Here's how the part is built. I have some questions about the finished solid (model axes, mm). Round coordinates to 2 decimals unless told otherwise and drop trailing zeros. Write each loop counter-clockwise with the first axis right and the second up, starting at its lowest first coordinate (ties: lowest second). Pieces come first, ordered by that corner, then holes. Notation, with made-up numbers: (41, 26.25) - (97, 26.25) arc R22 cw to (97, 50.25) - close; hole circle Ø10 at (-28, 4). An arc over 180 degrees is marked (long way). Return JSON: item names as keys, results as strings. Group by question number.
```python
from build123d import *

# Parameters (mm, degrees)
SKETCH_1_W          = 30
SKETCH_1_H          = 30
EXTRUDE_1_DEPTH     = 10
SKETCH_2_R          = 1.5
CUT_EXTRUDE_1_DEPTH = 11
FILLET_1_R          = 1
SKETCH_3_R          = 14
CUT_EXTRUDE_2_DEPTH = 11


with BuildPart() as part:
    # 草图1 → 凸台-拉伸1 (new body)
    with BuildSketch(Plane(origin=(0, 0, 0), x_dir=(1, 0, 0), z_dir=(0, 1, 0))):
        Rectangle(SKETCH_1_W, SKETCH_1_H)
    extrude(amount=EXTRUDE_1_DEPTH)

    # 草图2 → 切除-拉伸1 (cut, through all)
    with BuildSketch(Plane(origin=(0, 10, 0), x_dir=(1, 0, 0), z_dir=(0, 1, 0))):
        with Locations((-12.3, 12.3)):
            Circle(SKETCH_2_R)
        with Locations((12.3, 12.3)):
            Circle(SKETCH_2_R)
        with Locations((-12.3, -12.3)):
            Circle(SKETCH_2_R)
        with Locations((12.3, -12.3)):
            Circle(SKETCH_2_R)
    extrude(amount=-CUT_EXTRUDE_1_DEPTH, mode=Mode.SUBTRACT)

    # 圆角1
    fillet_1_edges = [part.edges().sort_by_distance(p)[0] for p in [
        (15, 5, 15),
        (-15, 5, 15),
        (-15, 5, -15),
        (15, 5, -15),
    ]]
    fillet(fillet_1_edges, radius=FILLET_1_R)

    # 草图3 → 切除-拉伸2 (cut, through all)
    with BuildSketch(Plane(origin=(0, 10, 0), x_dir=(1, 0, 0), z_dir=(0, 1, 0))):
        Circle(SKETCH_3_R)
    extrude(amount=-CUT_EXTRUDE_2_DEPTH, mode=Mode.SUBTRACT)


solid = part.part
```
1) If we mould it in two halves opening along X, with no side actions, what happens to faces 1 (the cylindrical face through (13.686, 5.07, -11.725)), 2 (the flat face through (0, 5, 15)), 3 (the flat face through (15, 5, 0))? For each: released by +X, released by -X, zero draft, split by the parting line, or undercut.
2) Imagine slicing it at A-A (x = 0). Please give me the cut outline in (y, z).
3) Imagine slicing it at D-D (x = -12.3). Please give me the cut outline in (y, z), plus the area to 3 significant figures.
4) Imagine slicing it at C-C (y = 1.5). Please give me the cut outline in (x, z), plus the area to 3 significant figures.
5) Will this pin go through, and if not, where does the flat tip stop? pin 1 Ø4 at (x, z) = (-12.3, -12.3) entering from +Y.
6) Imagine slicing it at B-B (z = 0). Please give me the cut outline in (x, y).
7) I need wall thicknesses on line 1 along X through (y, z) = (6, -11.75); line 2 along X through (y, z) = (5.5, 12); line 3 along Z through (x, y) = (0, 2.75). Which ranges of each line are inside material? Lowest first, please.
Results found:
{
 "1": {"face 1": "undercut", "face 2": "zero draft", "face 3": "released by +X"},
 "2": {"outline": "(0, -15) - (10, -15) - (10, -14) - (0, -14) - close; (0, 14) - (10, 14) - (10, 15) - (0, 15) - close"},
 "3": {"outline": "(0, -15) - (10, -15) - (10, -13.8) - (0, -13.8) - close; (0, -10.8) - (10, -10.8) - (10, -6.69) - (0, -6.69) - close; (0, 6.69) - (10, 6.69) - (10, 10.8) - (0, 10.8) - close; (0, 13.8) - (10, 13.8) - (10, 15) - (0, 15) - close", "area": "106 mm²"},
 "4": {"outline": "(-15, -14) arc R1 ccw to (-14, -15) - (14, -15) arc R1 ccw to (15, -14) - (15, 14) arc R1 ccw to (14, 15) - (-14, 15) arc R1 ccw to (-15, 14) - close; hole circle Ø28 at (0, 0); hole circle Ø3 at (-12.3, -12.3); hole circle Ø3 at (-12.3, 12.3); hole circle Ø3 at (12.3, -12.3); hole circle Ø3 at (12.3, 12.3)", "area": "255 mm²"},
 "5": {"pin 1": "stops at y = 10"},
 "6": {"outline": "(-15, 0) - (-14, 0) - (-14, 10) - (-15, 10) - close; (14, 0) - (15, 0) - (15, 10) - (14, 10) - close"},
 "7": {"line 1": "x = -15 to -13.7, -10.9 to -7.61, 7.61 to 10.9, 13.7 to 15", "line 2": "x = -15 to -13.77, -10.83 to -7.21, 7.21 to 10.83, 13.77 to 15", "line 3": "z = -15 to -14, 14 to 15"}
}
